Can you work these out from the model? Positions are in its coordinate system, mm. A direction names the side the tool comes from. Coordinates: 2 decimals unless noted, no trailing zeros. Loops run counter-clockwise (first coordinate to the right, second up) from the corner with the lowest first, then second, coordinate; pieces in that order, holes last.
```python
from build123d import *

# Parameters (mm, degrees)
F1_DEPTH = 6


with BuildPart() as f1:
    # F0 (on Top) → F1 (new body)
    with BuildSketch(Plane.XY):
        with BuildLine():
            Line((3.66008, 29.904429), (-3.66008, 29.904429))
            ThreePointArc((-3.66008, 29.904429), (-4.773266, 29.566), (-5.509717, 28.665246))
            Line((-5.509717, 28.665246), (-12.904586, 10.687453))
            ThreePointArc((-12.904586, 10.687453), (-12.954508, 10.083702), (-12.646693, 9.56192))
            ThreePointArc((-12.646693, 9.56192), (-12.248494, 7.071671), (-14.604212, 6.171398))
            ThreePointArc((-14.604212, 6.171398), (-15.209996, 6.177082), (-15.707898, 5.831973))
            Line((-15.707898, 5.831973), (-27.57969, -9.561068))
            ThreePointArc((-27.57969, -9.561068), (-27.99154, -10.64923), (-27.728035, -11.782492))
            Line((-27.728035, -11.782492), (-24.067955, -18.121937))
            ThreePointArc((-24.067955, -18.121937), (-23.218274, -18.916769), (-22.069973, -19.104178))
            Line((-22.069973, -19.104178), (-2.803313, -16.519426))
            ThreePointArc((-2.803313, -16.519426), (-2.255488, -16.260784), (-1.957519, -15.733317))
            ThreePointArc((-1.957519, -15.733317), (0, -14.143342), (1.957519, -15.733317))
            ThreePointArc((1.957519, -15.733317), (2.255488, -16.260784), (2.803313, -16.519426))
            Line((2.803313, -16.519426), (22.069973, -19.104178))
            ThreePointArc((22.069973, -19.104178), (23.218274, -18.916769), (24.067955, -18.121937))
            Line((24.067955, -18.121937), (27.728035, -11.782492))
            ThreePointArc((27.728035, -11.782492), (27.99154, -10.64923), (27.57969, -9.561068))
            Line((27.57969, -9.561068), (15.707898, 5.831973))
            ThreePointArc((15.707898, 5.831973), (15.209996, 6.177082), (14.604212, 6.171398))
            ThreePointArc((14.604212, 6.171398), (12.248494, 7.071671), (12.646693, 9.56192))
            ThreePointArc((12.646693, 9.56192), (12.954508, 10.083702), (12.904586, 10.687453))
            Line((12.904586, 10.687453), (5.509717, 28.665246))
            ThreePointArc((5.509717, 28.665246), (4.773266, 29.566), (3.66008, 29.904429))
        make_face()
        with BuildLine():
            ThreePointArc((-10.180424, -4.16641), (-9.526279, 5.5), (-1.481994, 10.899711))
            ThreePointArc((-1.481994, 10.899711), (-1.17274, 11.066276), (-1.049358, 11.395152))
            Line((-1.049358, 11.395152), (-1.049358, 13.410798))
            ThreePointArc((-1.049358, 13.410798), (-1.216711, 13.784088), (-1.606741, 13.907494))
            ThreePointArc((-1.606741, 13.907494), (-3.955309, 13.429651), (-6.187959, 12.558231))
            ThreePointArc((-6.187959, 12.558231), (-8.437578, 12.891077), (-8.92159, 15.113082))
            Line((-8.92159, 15.113082), (-5.437741, 23.582728))
            ThreePointArc((-5.437741, 23.582728), (-4.701289, 24.483481), (-3.588104, 24.82191))
            Line((-3.588104, 24.82191), (3.588104, 24.82191))
            ThreePointArc((3.588104, 24.82191), (4.701289, 24.483481), (5.437741, 23.582728))
            Line((5.437741, 23.582728), (8.92159, 15.113082))
            ThreePointArc((8.92159, 15.113082), (8.437578, 12.891077), (6.187959, 12.558231))
            ThreePointArc((6.187959, 12.558231), (3.955309, 13.429651), (1.606741, 13.907494))
            ThreePointArc((1.606741, 13.907494), (1.216711, 13.784088), (1.049358, 13.410798))
            Line((1.049358, 13.410798), (1.049358, 11.395152))
            ThreePointArc((1.049358, 11.395152), (1.17274, 11.066276), (1.481994, 10.899711))
            ThreePointArc((1.481994, 10.899711), (9.526279, 5.5), (10.180424, -4.16641))
            ThreePointArc((10.180424, -4.16641), (10.170047, -4.517515), (10.39317, -4.788805))
            Line((10.39317, -4.788805), (12.13877, -5.796628))
            ThreePointArc((12.13877, -5.796628), (12.545726, -5.838342), (12.847614, -5.562268))
            ThreePointArc((12.847614, -5.562268), (13.608073, -3.289428), (13.969726, -0.920186))
            ThreePointArc((13.969726, -0.920186), (15.382789, 0.861619), (17.549107, 0.169783))
            Line((17.549107, 0.169783), (23.142112, -7.082143))
            ThreePointArc((23.142112, -7.082143), (23.553962, -8.170305), (23.290457, -9.303566))
            Line((23.290457, -9.303566), (19.702353, -15.518344))
            ThreePointArc((19.702353, -15.518344), (18.852672, -16.313177), (17.704371, -16.500586))
            Line((17.704371, -16.500586), (8.627518, -15.282864))
            ThreePointArc((8.627518, -15.282864), (6.945211, -13.752695), (7.781768, -11.638045))
            ThreePointArc((7.781768, -11.638045), (9.652765, -10.140223), (11.240872, -8.345226))
            ThreePointArc((11.240872, -8.345226), (11.329015, -7.945747), (11.089412, -7.614169))
            Line((11.089412, -7.614169), (9.343812, -6.606347))
            ThreePointArc((9.343812, -6.606347), (8.997306, -6.548761), (8.698429, -6.7333))
            ThreePointArc((8.698429, -6.7333), (0, -11), (-8.698429, -6.7333))
            ThreePointArc((-8.698429, -6.7333), (-8.997306, -6.548761), (-9.343812, -6.606347))
            Line((-9.343812, -6.606347), (-11.089412, -7.614169))
            ThreePointArc((-11.089412, -7.614169), (-11.329015, -7.945747), (-11.240872, -8.345226))
            ThreePointArc((-11.240872, -8.345226), (-9.652765, -10.140223), (-7.781768, -11.638045))
            ThreePointArc((-7.781768, -11.638045), (-6.945211, -13.752695), (-8.627518, -15.282864))
            Line((-8.627518, -15.282864), (-17.704371, -16.500586))
            ThreePointArc((-17.704371, -16.500586), (-18.852672, -16.313177), (-19.702353, -15.518344))
            Line((-19.702353, -15.518344), (-23.290457, -9.303566))
            ThreePointArc((-23.290457, -9.303566), (-23.553962, -8.170305), (-23.142112, -7.082143))
            Line((-23.142112, -7.082143), (-17.549107, 0.169783))
            ThreePointArc((-17.549107, 0.169783), (-15.382789, 0.861619), (-13.969726, -0.920186))
            ThreePointArc((-13.969726, -0.920186), (-13.608073, -3.289428), (-12.847614, -5.562268))
            ThreePointArc((-12.847614, -5.562268), (-12.545726, -5.838342), (-12.13877, -5.796628))
            Line((-12.13877, -5.796628), (-10.39317, -4.788805))
            ThreePointArc((-10.39317, -4.788805), (-10.170047, -4.517515), (-10.180424, -4.16641))
        make_face(mode=Mode.SUBTRACT)
    extrude(amount=F1_DEPTH)


solid = f1.part
```
(1) If we mould it in two halves opening along X, with no side actions, what happens to faces 3 (the flat face through (-21.561, -1.757, 2.958)), 4 (the cylindrical face through (-8.413, 12.868, 2.958)), 5 (the flat face through (12.302, -17.794, 2.958)), 6 (the flat face through (2, -11, 0))? For each: released by +X, released by -X, zero draft, split by the parting line, or undercut.
Check values:
face 3: released by -X
face 4: undercut
face 5: undercut
face 6: zero draft
(2) I want a section at C-C on y = -12.5. Write out the boundary of the cut face in (x, z) (3 decimals), then the cut area to 3 significant figures.
Check values:
outline: (-27.314, 0) - (-21.445, 0) - (-21.445, 6) - (-27.314, 6) - close; (-7.061, 0) - (7.061, 0) - (7.061, 6) - (-7.061, 6) - close; (21.445, 0) - (27.314, 0) - (27.314, 6) - (21.445, 6) - close
area: 155 mm2
(3) I want a section at A-A on x = 18.5. Write out the boundary of the cut face in (y, z), then the cut area to 3 significant figures.
Check values:
outline: (-18.63, 0) - (-16.45, 0) - (-16.45, 6) - (-18.63, 6) - close; (-1.06, 0) - (2.21, 0) - (2.21, 6) - (-1.06, 6) - close
area: 32.7 mm2
(4) I want a section at D-D on y = -2.5. Write out the boundary of the cut face in (x, z).
Check values:
outline: (-22.13, 0) - (-19.61, 0) - (-19.61, 6) - (-22.13, 6) - close; (-13.77, 0) - (-10.71, 0) - (-10.71, 6) - (-13.77, 6) - close; (10.71, 0) - (13.77, 0) - (13.77, 6) - (10.71, 6) - close; (19.61, 0) - (22.13, 0) - (22.13, 6) - (19.61, 6) - close
(5) I'm going to push flat-ended pins straight in: pin 1 (1 mm diameter, centred on y = 19.5, z = 1, fed in from -X); pin 2 (0.6 mm diameter, centred on y = 12.5, z = 4, fed in from +X); pin 3 (1 mm diameter, centred on y = 12.5, z = 4, fed in from -X). Where does each tip first touch, or does it pass through?
Check values:
pin 1: stops at x = -9.49
pin 2: stops at x = 12.28
pin 3: stops at x = -12.36
(6) Which directions (+Z, -Z, +X, -X, +Y, -Y) give clear straight access to the entire face, cutting with the end or side of a thin tool? Please do faces 1 (the cylindrical face through (-27.99, -10.63, 2.96)), 2 (the flat face through (11.254, -5.286, 2.958)).
Check values:
face 1: +Z, -Z, -X
face 2: +Z, -Z
(7) If I drill on probe 1 along X at (y, z) = (-0.5, 2.6); probe 2 along Y at (x, z) = (-10, 2.45); probe 3 along Y at (x, z) = (-5, 3.15), over which ranges is the centre line in solid material (lowest first)?
Check values:
probe 1: x = -20.59 to -18.07, -14.04 to -10.99, 10.99 to 14.04, 18.07 to 20.59
probe 2: y = -17.48 to -15.47, -9.8 to -6.99, 4.58 to 17.75
probe 3: y = -16.81 to -9.8, 9.8 to 13.08, 24.24 to 29.39
(8) I want a section at B-B on y = 8.5. Write out the boundary of the cut face in (x, z), then the cut area to 3 significant figures.
Check values:
outline: (-12.03, 0) - (-6.98, 0) - (-6.98, 6) - (-12.03, 6) - close; (6.98, 0) - (12.03, 0) - (12.03, 6) - (6.98, 6) - close
area: 60.5 mm2
